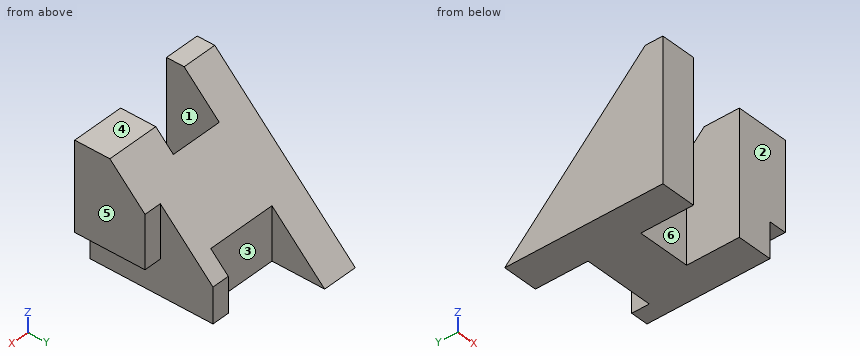
```python
from build123d import *

# Parameters (mm, degrees)
SKETCH1_W           = 8
SKETCH1_H           = 9
BOSS_EXTRUDE1_DEPTH = 8
SKETCH2_W           = 4
SKETCH2_H           = 3
CUT_EXTRUDE1_DEPTH  = 3
SKETCH3_W           = 2
SKETCH3_H           = 2
CUT_EXTRUDE2_DEPTH  = 2
CUT_EXTRUDE3_DEPTH  = 1
CUT_EXTRUDE4_DEPTH  = 9
SKETCH6_W           = 3
SKETCH6_H           = 3
CUT_EXTRUDE5_DEPTH  = 9
SKETCH7_W           = 3
SKETCH7_H           = 1
CUT_EXTRUDE6_DEPTH  = 2


with BuildPart() as part:
    # Sketch1 → Boss-Extrude1 (new body)
    with BuildSketch(Plane.XY):
        Rectangle(SKETCH1_W, SKETCH1_H)
    extrude(amount=BOSS_EXTRUDE1_DEPTH)

    # Sketch2 → Cut-Extrude1 (cut)
    with BuildSketch(Plane(origin=(0, 4.5, 0), x_dir=(1, 0, 0), z_dir=(0, 1, 0))):
        with Locations((0, -1.5)):
            Rectangle(SKETCH2_W, SKETCH2_H)
    extrude(amount=-CUT_EXTRUDE1_DEPTH, mode=Mode.SUBTRACT)

    # Sketch3 → Cut-Extrude2 (cut)
    with BuildSketch(Plane(origin=(0, 4.5, 0), x_dir=(1, 0, 0), z_dir=(0, 1, 0))):
        with Locations((3, -1)):
            Rectangle(SKETCH3_W, SKETCH3_H)
    extrude(amount=-CUT_EXTRUDE2_DEPTH, mode=Mode.SUBTRACT)

    # Sketch4 → Cut-Extrude3 (cut)
    with BuildSketch(Plane(origin=(4, 0, 0), x_dir=(0, 0, -1), z_dir=(1, 0, 0))):
        Polygon((0, -4.5), (0, 2.5), (-2, 2.5), (-5, -0.5), (-2, -0.5), (-2, -4.5), align=None)
    extrude(amount=-CUT_EXTRUDE3_DEPTH, mode=Mode.SUBTRACT)

    # Sketch5 → Cut-Extrude4 (cut, through all)
    with BuildSketch(Plane(origin=(4, 0, 0), x_dir=(0, 0, -1), z_dir=(1, 0, 0))):
        Polygon((0, 4.5), (-8, -3.5), (-8, 4.5), align=None)
    extrude(amount=-CUT_EXTRUDE4_DEPTH, mode=Mode.SUBTRACT)

    # Sketch6 → Cut-Extrude5 (cut, through all)
    with BuildSketch(Plane(origin=(0, 0, 0), x_dir=(-1, 0, 0), z_dir=(0, 0, -1))):
        with Locations((0.5, -3)):
            Rectangle(SKETCH6_W, SKETCH6_H)
    extrude(amount=-CUT_EXTRUDE5_DEPTH, mode=Mode.SUBTRACT)

    # Sketch7 → Cut-Extrude6 (cut)
    with BuildSketch(Plane.XZ.offset(4.5)):
        with Locations((2.5, 7.5)):
            Rectangle(SKETCH7_W, SKETCH7_H)
    extrude(amount=-CUT_EXTRUDE6_DEPTH, mode=Mode.SUBTRACT)


solid = part.part
```
Verification items for the finished model (mm, model axes). Face numbers are marked on the shaded views. A direction names the side the tool comes from. Give positions to 0.01 mm unless a question says otherwise; leave off trailing zeros. Order: outer loops, then holes, each group sorted by start corner. A loop starts at its lowest first (then second) coordinate and runs counter-clockwise, first axis right, second up. Notation, with made-up numbers: M 42.25,-3 L 88.25,-3 A25 ccw 88.25,29 Z; hole C -10.5,37.25 d3. An arc over 180 degrees is marked long. Return JSON: item names as keys, results as strings. Group by question number.
1) Section check B-B on z = 6.5. Record the cut outline in (x, y), and give its area (3 significant figures).
2) Go/stop test with flat-tipped pins: pin 1 Ø0.5 at (x, z) = (3.5, 3.5) entering from +Y; pin 2 Ø3.5 at (x, z) = (0.5, 1.5) entering from +Y; pin 3 Ø1.5 at (y, z) = (3, 5) entering from -X; pin 4 Ø2 at (x, y) = (2.5, -3.5) entering from +Z. Record where each tip stops, or that it passes through.
3) Section check D-D on y = -1.75. Record the cut outline in (x, z).
4) Mould release check, pull along X, two halves, no side actions. Record for the marked faces 4, 5 and 6: pulls with the +X half, pulls with the -X half, needs draft (parallel to the pull), parting line crosses it, or undercut.
5) Scan lines: line 1 (X direction, y = -2, z = 4); line 2 (X direction, y = -2, z = 1.75); line 3 (Y direction, x = -2.5, z = 1.5). Record each from-to range of solid material in increasing order.
6) Section check A-A on y = 2.25. Record the cut outline in (x, z), and give its area (3 significant figures).
7) Section check C-C on z = 2.5. Record the cut outline in (x, y), and give its area (3 significant figures).
8) Access from +Z, -Z, +X, -X, +Y, -Y to the whole of each face (thin tool, end or side, straight path). Record for the marked faces 1, 2 and 3.
Answer block:
{
 "1": {"outline": "M -4,-4.5 L -2,-4.5 L -2,-2 L -4,-2 Z; M 1,-4.5 L 4,-4.5 L 4,-2 L 1,-2 Z", "area": "12.5 mm^2"},
 "2": {"pin 1": "stops at y = -0.5", "pin 2": "stops at y = 2.5", "pin 3": "passes through", "pin 4": "stops at z = 7"},
 "3": {"outline": "M -4,0 L -2,0 L -2,6.25 L -4,6.25 Z; M 1,0 L 3,0 L 3,2 L 4,2 L 4,6.25 L 1,6.25 Z"},
 "4": {"face 4": "needs draft", "face 5": "pulls with the +X half", "face 6": "undercut"},
 "5": {"line 1": "x = -4 to -2, 1 to 4", "line 2": "x = -4 to -2, 1 to 3", "line 3": "y = -4.5 to 3"},
 "6": {"outline": "M -4,0 L -2,0 L -2,2.25 L -4,2.25 Z; M 2,0 L 3,0 L 3,2.25 L 2,2.25 Z", "area": "6.75 mm^2"},
 "7": {"outline": "M -4,-4.5 L -2,-4.5 L -2,-1.5 L 1,-1.5 L 1,-4.5 L 4,-4.5 L 4,-0.5 L 3,-0.5 L 3,2 L 2,2 L 2,1.5 L -2,1.5 L -2,2 L -4,2 Z", "area": "38.5 mm^2"},
 "8": {"face 1": "+Z, -Z, -Y", "face 2": "+Z, -Z, +X, -X, -Y", "face 3": "+Z, -Z, +Y"}
}
